from build123d import *

# Parameters (mm, degrees)
F1_DEPTH = 4
F3_DEPTH = 1.5
F5_DEPTH = 1.5
F6_R     = 2.5
F7_DEPTH = 25
F9_DEPTH = 1.5


with BuildPart() as f1:
    # F0 (on Top) → F1 (new body)
    with BuildSketch(Plane.XY):
        with BuildLine():
            ThreePointArc((12.5, 25), (0, 12.5), (12.5, 0))
            Line((12.5, 0), (59.5057010651, 0))
            ThreePointArc((59.5057010651, 0), (72.0057010651, 12.5), (59.5057010651, 25))
            Line((59.5057010651, 25), (12.5, 25))
        make_face()
    extrude(amount=F1_DEPTH)

    # F2 (on face) → F3 (cut)
    with BuildSketch(Plane.XY.offset(4)):
        with BuildLine():
            Line((59.5057010651, 22.5), (12.5, 22.5))
            ThreePointArc((12.5, 22.5), (2.5, 12.5), (12.5, 2.5))
            Line((12.5, 2.5), (59.5057010651, 2.5))
            ThreePointArc((59.5057010651, 2.5), (69.5057010651, 12.5), (59.5057010651, 22.5))
        make_face()
    extrude(amount=-F3_DEPTH, mode=Mode.SUBTRACT)

    # F4 (on face) → F5 (join)
    with BuildSketch(Plane.XY.offset(2.5)):
        with BuildLine():
            ThreePointArc((3.4807692308, 8.1810329555), (8.4903660528, 8.1643250902), (11, 12.5))
            ThreePointArc((11, 12.5), (8.4903660528, 16.8356749098), (3.4807692308, 16.8189670445))
            ThreePointArc((3.4807692308, 16.8189670445), (2.5, 12.5), (3.4807692308, 8.1810329555))
        make_face()
    extrude(amount=F5_DEPTH)

    # F6 (on face) → F7 (cut)
    with BuildSketch(Plane.XY.offset(4)):
        with Locations((6, 12.5)):
            Circle(F6_R)
    extrude(amount=-F7_DEPTH, mode=Mode.SUBTRACT)

    # F8 (on face) → F9 (join)
    with BuildSketch(Plane.XY.offset(2.5)):
        with BuildLine():
            Line((51.5800477753, 23.6497587322), (51.5800477753, 29.9388212322))
            Line((51.5800477753, 29.9388212322), (21.8339540253, 29.9388212322))
            Line((21.8339540253, 29.9388212322), (21.8339540253, 24.7695503988))
            Line((21.8339540253, 24.7695503988), (23.6409601852, 22.5))
            Line((23.6409601852, 22.5), (29.7308289031, 22.5))
            add(Edge.make_bspline(
                [(28.4485373586, 23.8125191488), (29.2209345705, 23.0401219369), (29.7308289031, 22.5)],
                knots=[0, 0, 0, 0.4943342156, 0.4943342156, 0.4943342156], degree=2))
            Line((28.4485373586, 23.8125191488), (31.5409852753, 23.7148628988))
            Line((31.5409852753, 23.7148628988), (34.3665061086, 23.6497587322))
            Line((34.3665061086, 23.6497587322), (51.5800477753, 23.6497587322))
        make_face()
    extrude(amount=F9_DEPTH)


solid = f1.part
For this review, take the finished solid that the model builds, in its own axes (mm). A direction names the side the tool comes from. Round coordinates to 2 decimals unless told otherwise and drop trailing zeros. Order: outer loops, then holes, each group sorted by start corner. A loop starts at its lowest first (then second) coordinate and runs counter-clockwise, first axis right, second up. Notation, with made-up numbers: M 21,-39.5 L 52,-39.5 A22 ccw 52,-16.5 Z; hole C -33,21.25 d11. An arc over 180 degrees is marked long. Use a Markdown table: item, result. Add a question column.
Item 1: Add section C-C, the plane z = 1.2. Give the boundary of the cut face in (x, y), then the cut area to 3 significant figures.
Item 2: Insertion check: pin 1 (2 mm diameter, centred on y = 7.5, z = 1, fed in from -X); pin 2 (1.5 mm diameter, centred on x = 54.5, y = 21, fed in from +Z); pin 3 (0.8 mm diameter, centred on y = 27.5, z = 3, fed in from +X); pin 4 (4.5 mm diameter, centred on x = 6, y = 12.5, fed in from -Z). Each pin has a flat end and moves straight along its axis. Give the tip position at first contact, or say it passes through.
Item 3: Add section D-D, the plane y = 3.75. Give the boundary of the cut face in (x, z), then the cut area to 3 significant figures.
Item 4: Mouldability with a two-part tool opening along X and no side actions: class faces 4 (the flat face through (33, 23, 4)), 5 (the flat face through (51.58, 27, 3)), 6 (the cylindrical face through (7.15, 10.28, 2.03)) as released by +X, released by -X, zero draft, split by the parting line, or undercut.
Item 5: Add section B-B, the plane y = 11. Give the boundary of the cut face in (x, z), then the cut area to 3 significant figures.
Item 6: To check wall thickness, follow line 1 along X through (y, z) = (14.5, 3.5); line 2 along Y through (x, z) = (39.5, 2.7); line 3 along Y through (x, z) = (21, 3.25). State the ranges of each line that lie inside material, in increasing order.
Item 7: Tool access review of faces 1 (the flat face through (36, 22.5, 3)), 2 (the flat face through (36, 28, 2.5)), 3 (the flat face through (21.834, 28, 3)): name each direction out of +Z, -Z, +X, -X, +Y, -Y from which nothing blocks a thin tool from reaching the whole face with its end or side.
Item 8: Add section A-A, the plane x = 45.5. Give the boundary of the cut face in (y, z), then the cut area to 3 significant figures.
Geometry results:
| question | item | result |
|---|---|---|
| 1 | outline | M 12.5,0 L 59.51,0 A12.5 ccw 59.51,25 L 12.5,25 A12.5 ccw Z; hole C 6,12.5 d5 |
| 1 | area | 1,650 mm² |
| 2 | pin 1 | stops at x = 0.66 |
| 2 | pin 2 | stops at z = 2.5 |
| 2 | pin 3 | stops at x = 51.58 |
| 2 | pin 4 | passes through |
| 3 | outline | M 3.57,0 L 68.43,0 L 68.43,4 L 64.35,4 L 64.35,2.5 L 7.66,2.5 L 7.66,4 L 3.57,4 Z |
| 3 | area | 174 mm² |
| 4 | face 4 | zero draft |
| 4 | face 5 | released by +X |
| 4 | face 6 | undercut |
| 5 | outline | M 0.09,0 L 4,0 L 4,4 L 0.09,4 Z; M 8,0 L 71.92,0 L 71.92,4 L 69.39,4 L 69.39,2.5 L 10.77,2.5 L 10.77,4 L 8,4 Z |
| 5 | area | 183 mm² |
| 6 | line 1 | x = 0.16 to 4.5, 7.5 to 10.58, 69.3 to 71.84 |
| 6 | line 2 | y = 0 to 2.5, 22.5 to 29.94 |
| 6 | line 3 | y = 0 to 2.5, 22.5 to 25 |
| 7 | face 1 | +Z |
| 7 | face 2 | -Z, +X, -X, +Y |
| 7 | face 3 | +Z, -Z, -X, +Y |
| 8 | outline | M 0,0 L 25,0 L 25,2.5 L 29.94,2.5 L 29.94,4 L 22.5,4 L 22.5,2.5 L 2.5,2.5 L 2.5,4 L 0,4 Z |
| 8 | area | 77.4 mm² |
